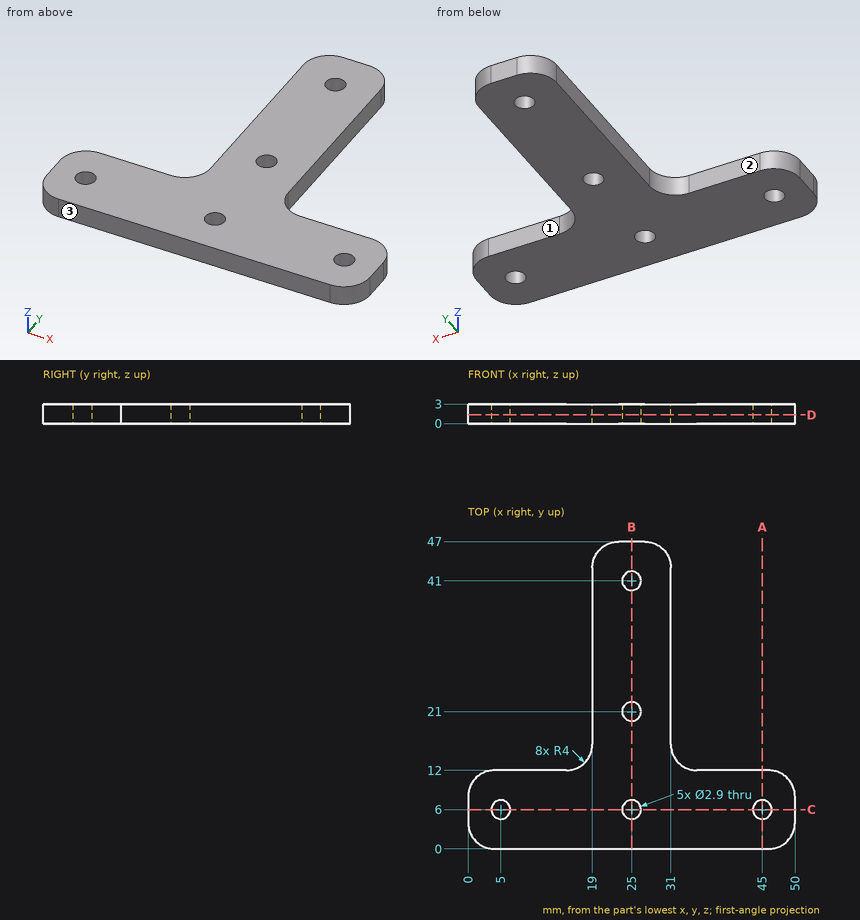
Part print with two shaded views. Sizes in mm from the minimum x, y, z corner. A direction names the side the tool comes from. Coordinates: 2 decimals unless noted, no trailing zeros. Loops run counter-clockwise (first coordinate to the right, second up) from the corner with the lowest first, then second, coordinate; pieces in that order, holes last. Notation, with made-up numbers: (11, -9.5) - (35, -9.5) arc R21 cw to (35, 21.5) - close; hole circle Ø1 at (72.5, -22.5). An arc over 180 degrees is marked (long way). Write each question's results on one line, items separated by ' | '. Start each with the question number.
Q1. Which spindle directions (+Z, -Z, +X, -X, +Y, -Y) get a long thin tool onto all of the face, cutting with end or side? Do the marked faces 1, 2 and 3. Say none if no direction does.
Q2. Slice it at B-B on x = 25. Give the cut face in (y, z), and give its area (3 significant figures).
Q3. Slice it at D-D on z = 1.35. Give the cut face in (x, y).
Q4. Slice it at C-C on y = 6. Give the cut face in (x, z), and give its area (3 significant figures).
Q5. Drop a flat-ended pin along its axis: pin 1 Ø1.5 at (y, z) = (23, 2) entering from +X. Give the stop position or say it passes through.
Q6. Slice it at A-A on x = 45. Give the cut face in (y, z).
Q7. Probe line 1 along Y through (x, z) = (25, 0.7); line 2 along Y through (x, z) = (5, 1.15); line 3 along X through (y, z) = (27.5, 0.8). List the from-to ranges inside material, lowest first.
Answer:
1) face 1: +Z, -Z, +X, +Y | face 2: +Z, -Z, -X, +Y | face 3: +Z, -Z, +X, -X, -Y
2) outline: (0, 0) - (4.55, 0) - (4.55, 3) - (0, 3) - close; (7.45, 0) - (19.55, 0) - (19.55, 3) - (7.45, 3) - close; (22.45, 0) - (39.55, 0) - (39.55, 3) - (22.45, 3) - close; (42.45, 0) - (47, 0) - (47, 3) - (42.45, 3) - close | area: 115 mm2
3) outline: (0, 4) arc R4 ccw to (4, 0) - (46, 0) arc R4 ccw to (50, 4) - (50, 8) arc R4 ccw to (46, 12) - (35, 12) arc R4 cw to (31, 16) - (31, 43) arc R4 ccw to (27, 47) - (23, 47) arc R4 ccw to (19, 43) - (19, 16) arc R4 cw to (15, 12) - (4, 12) arc R4 ccw to (0, 8) - close; hole circle Ø2.9 at (5, 6); hole circle Ø2.9 at (25, 6); hole circle Ø2.9 at (25, 21); hole circle Ø2.9 at (25, 41); hole circle Ø2.9 at (45, 6)
4) outline: (0, 0) - (3.55, 0) - (3.55, 3) - (0, 3) - close; (6.45, 0) - (23.55, 0) - (23.55, 3) - (6.45, 3) - close; (26.45, 0) - (43.55, 0) - (43.55, 3) - (26.45, 3) - close; (46.45, 0) - (50, 0) - (50, 3) - (46.45, 3) - close | area: 124 mm2
5) pin 1: stops at x = 31
6) outline: (0, 0) - (4.55, 0) - (4.55, 3) - (0, 3) - close; (7.45, 0) - (12, 0) - (12, 3) - (7.45, 3) - close
7) line 1: y = 0 to 4.55, 7.45 to 19.55, 22.45 to 39.55, 42.45 to 47 | line 2: y = 0 to 4.55, 7.45 to 12 | line 3: x = 19 to 31
